For this review, take the finished solid that the model builds, in its own axes (mm). Coordinates: 2 decimals unless noted, no trailing zeros. Loops run counter-clockwise (first coordinate to the right, second up) from the corner with the lowest first, then second, coordinate; pieces in that order, holes last.
```python
from build123d import *

# Parameters (mm, degrees)
SKETCH1_R           = 3.75
BOSS_EXTRUDE1_DEPTH = 1
SKETCH2_R           = 2
CUT_EXTRUDE3_DEPTH  = 1
SKETCH3_W           = 2
SKETCH3_H           = 1
SKETCH3_W_2         = 1
SKETCH3_H_2         = 2
CUT_EXTRUDE4_DEPTH  = 1


with BuildPart() as part:
    # Sketch1 → Boss-Extrude1 (new body)
    with BuildSketch(Plane.XY):
        Circle(SKETCH1_R)
        with Locations((7, 0)):
            Circle(SKETCH1_R)
    extrude(amount=BOSS_EXTRUDE1_DEPTH)

    # Sketch2 → Cut-Extrude3 (cut)
    with BuildSketch(Plane.XY):
        Circle(SKETCH2_R)
        with Locations((6.883478598, 0)):
            Circle(SKETCH2_R)
    extrude(amount=CUT_EXTRUDE3_DEPTH, mode=Mode.SUBTRACT)

    # Sketch3 → Cut-Extrude4 (cut)
    with BuildSketch(Plane.XY):
        with Locations((7, -2.86532029)):
            Rectangle(SKETCH3_W, SKETCH3_H)
        with Locations((9.86532029, 0)):
            Rectangle(SKETCH3_W_2, SKETCH3_H_2)
        with Locations((7, 2.86532029)):
            Rectangle(SKETCH3_W, SKETCH3_H)
        with Locations((-0.095382463, -2.86532029)):
            Rectangle(SKETCH3_W, SKETCH3_H)
        with Locations((-0.095382463, 2.86532029)):
            Rectangle(SKETCH3_W, SKETCH3_H)
        with Locations((-2.960702753, 0)):
            Rectangle(SKETCH3_W_2, SKETCH3_H_2)
        with Locations((3.452308768, 0)):
            Rectangle(SKETCH3_W_2, SKETCH3_H_2)
    extrude(amount=CUT_EXTRUDE4_DEPTH, mode=Mode.SUBTRACT)


solid = part.part
```
Q1. Wall thickness on probe 1 along Y at (x, z) = (0, 0.45); probe 2 along Y at (x, z) = (0.5, 0.85); probe 3 along X at (y, z) = (2.5, 0.15): over which ranges is each line inside the solid? List them lowest first.
Q2. For pin 1 Ø1 at (x, y) = (4, 2) entering from -Z; pin 2 Ø0.5 at (x, z) = (0.5, 0.5) entering from -Y; pin 3 Ø0.5 at (y, z) = (3, 0.5) entering from -X, all flat-tipped, find the tip position at first contact; note any pin that passes through.
Q3. Consider section C-C (z = 0.45). Count the separate pieces of the cut face and the enclosed holes in it, then the cut area to 3 significant figures.
Q4. Consider section B-B (y = 0). State the section outline as (x, z) points, then the cut area to 3 significant figures.
Q5. The part is to be moulded in two halves that separate along Y. For faces 1 (the face through (8, 2.9, 0.5)), 2 (the face through (2.4, -0.3, 1)), say which applies: +Y half, -Y half, draft (parallel to the pull), parting line (faces both ways), or undercut.
Q6. Consider section A-A (x = 0). State the section outline as (y, z) points.
Q7. Consider section D-D (x = 8.5). State the section outline as (y, z) points, then the cut area to 3 significant figures.
Model answer:
1. probe 1: y = -3.75 to -3.37, -2.37 to -2, 2 to 2.37, 3.37 to 3.75
1. probe 2: y = -3.72 to -3.37, -2.37 to -1.94, 1.94 to 2.37, 3.37 to 3.72
1. probe 3: x = -2.8 to -1.1, 0.9 to 2.8, 4.2 to 6, 8 to 9.8
2. pin 1: stops at z = 0
2. pin 2: stops at y = -3.74
2. pin 3: stops at x = -2.55
3. separate pieces: 1
3. enclosed holes: 9
3. area: 48.3 mm2
4. outline: (-3.75, 0) - (-3.46, 0) - (-3.46, 1) - (-3.75, 1) - close; (-2.46, 0) - (-2, 0) - (-2, 1) - (-2.46, 1) - close; (2, 0) - (2.95, 0) - (2.95, 1) - (2, 1) - close; (3.95, 0) - (4.88, 0) - (4.88, 1) - (3.95, 1) - close; (8.88, 0) - (9.37, 0) - (9.37, 1) - (8.88, 1) - close; (10.37, 0) - (10.75, 0) - (10.75, 1) - (10.37, 1) - close
4. area: 3.50 mm2
5. face 1: undercut
5. face 2: draft
6. outline: (-3.75, 0) - (-3.37, 0) - (-3.37, 1) - (-3.75, 1) - close; (-2.37, 0) - (-2, 0) - (-2, 1) - (-2.37, 1) - close; (2, 0) - (2.37, 0) - (2.37, 1) - (2, 1) - close; (3.37, 0) - (3.75, 0) - (3.75, 1) - (3.37, 1) - close
7. outline: (-3.44, 0) - (-1.18, 0) - (-1.18, 1) - (-3.44, 1) - close; (1.18, 0) - (3.44, 0) - (3.44, 1) - (1.18, 1) - close
7. area: 4.52 mm2
